from build123d import *

# Parameters (mm, degrees)
F1_DEPTH = 4.7625
F2_R     = 5.08
F4_DEPTH = 4.7635


# Not quite as in the source:
# - a length typed as a fraction of an inch, garbled in the dataset ("3 / 203.2 mm" for 3/8 in), is restored


with BuildPart() as f1:
    # F0 (on Top) → F1 (new body)
    with BuildSketch(Plane.XY):
        Polygon((124.0544550598, 72.092982788), (-155.3455449402, 72.092982788), (-155.3455449402, 27.642982788), (-76.0003953454, 27.642982788), (-37.8705449402, -29.507017212), (-37.8705449402, -80.307017212), (6.5794550598, -80.307017212), (6.5794550598, -29.507017212), (44.7093054649, 27.642982788), (124.0544550598, 27.642982788), align=None)
    extrude(amount=F1_DEPTH)

    # F2
    f2_edges = [f1.edges().sort_by_distance(p)[0] for p in [
        (-155.345545, 27.642983, 2.38125),
        (-155.345545, 72.092983, 2.38125),
        (-37.870545, -80.307017, 2.38125),
        (6.579455, -80.307017, 2.38125),
        (-76.000395, 27.642983, 2.38125),
        (-37.870545, -29.507017, 2.38125),
        (6.579455, -29.507017, 2.38125),
        (44.709305, 27.642983, 2.38125),
        (124.054455, 27.642983, 2.38125),
        (124.054455, 72.092983, 2.38125),
    ]]
    fillet(f2_edges, radius=F2_R)

    # F3 (on face) → F4 (cut, through all)
    with BuildSketch(Plane.XY.offset(4.7625)):
        with BuildLine():
            Line((106.8459550598, 54.757482788), (97.5749550598, 54.757482788))
            ThreePointArc((97.5749550598, 54.757482788), (92.6854550598, 49.867982788), (97.5749550598, 44.978482788))
            Line((97.5749550598, 44.978482788), (106.8459550598, 44.978482788))
            ThreePointArc((106.8459550598, 44.978482788), (111.7354550598, 49.867982788), (106.8459550598, 54.757482788))
        make_face()
        with BuildLine():
            Line((33.6939550598, 54.757482788), (24.4229550598, 54.757482788))
            ThreePointArc((24.4229550598, 54.757482788), (19.5334550598, 49.867982788), (24.4229550598, 44.978482788))
            Line((24.4229550598, 44.978482788), (33.6939550598, 44.978482788))
            ThreePointArc((33.6939550598, 44.978482788), (38.5834550598, 49.867982788), (33.6939550598, 54.757482788))
        make_face()
        with BuildLine():
            ThreePointArc((-10.7560449402, -63.352517212), (-15.6455449402, -58.463017212), (-20.5350449402, -63.352517212))
            Line((-20.5350449402, -63.352517212), (-20.5350449402, -72.623517212))
            ThreePointArc((-20.5350449402, -72.623517212), (-15.6455449402, -77.513017212), (-10.7560449402, -72.623517212))
            Line((-10.7560449402, -72.623517212), (-10.7560449402, -63.352517212))
        make_face()
        with BuildLine():
            Line((-10.7560449402, 0.528482788), (-10.7560449402, 9.799482788))
            ThreePointArc((-10.7560449402, 9.799482788), (-15.6455449402, 14.688982788), (-20.5350449402, 9.799482788))
            Line((-20.5350449402, 9.799482788), (-20.5350449402, 0.528482788))
            ThreePointArc((-20.5350449402, 0.528482788), (-15.6455449402, -4.361017212), (-10.7560449402, 0.528482788))
        make_face()
        with BuildLine():
            Line((-128.8660449402, 54.757482788), (-138.1370449402, 54.757482788))
            ThreePointArc((-138.1370449402, 54.757482788), (-143.0265449402, 49.867982788), (-138.1370449402, 44.978482788))
            Line((-138.1370449402, 44.978482788), (-128.8660449402, 44.978482788))
            ThreePointArc((-128.8660449402, 44.978482788), (-123.9765449402, 49.867982788), (-128.8660449402, 54.757482788))
        make_face()
        with BuildLine():
            Line((-55.7140449402, 54.757482788), (-64.9850449402, 54.757482788))
            ThreePointArc((-64.9850449402, 54.757482788), (-69.8745449402, 49.867982788), (-64.9850449402, 44.978482788))
            Line((-64.9850449402, 44.978482788), (-55.7140449402, 44.978482788))
            ThreePointArc((-55.7140449402, 44.978482788), (-50.8245449402, 49.867982788), (-55.7140449402, 54.757482788))
        make_face()
    extrude(amount=-F4_DEPTH, mode=Mode.SUBTRACT)


solid = f1.part
Can you work these out from the model? Positions are in its coordinate system, mm. A direction names the side the tool comes from. Round coordinates to 2 decimals unless told otherwise and drop trailing zeros. Write each loop counter-clockwise with the first axis right and the second up, starting at its lowest first coordinate (ties: lowest second). Pieces come first, ordered by that corner, then holes. Notation, with made-up numbers: M 7,-25 L 41,-25 A15 cw 41,-3 Z; hole C 79.5,-23.5 d9. An arc over 180 degrees is marked long. Use a Markdown table: item, result.
Item 1: For pin 1 Ø2.5 at (x, z) = (-58.5, 1.5) entering from -Y; pin 2 Ø1.4 at (x, z) = (73, 3.5) entering from -Y; pin 3 Ø8 at (x, y) = (26, 56.5) entering from -Z; pin 4 Ø1.4 at (y, z) = (6, 2.5) entering from -X, each with a flat end and sliding along its axis, tell me the tip position at first contact or that it passes through.
Found:
| item | result |
|---|---|
| pin 1 | stops at y = -0.46 |
| pin 2 | stops at y = 27.64 |
| pin 3 | stops at z = 0 |
| pin 4 | stops at x = -62.03 |
Item 2: I want a section at C-C (z = 2.8). State how many separate pieces and enclosed holes the cut face has, and give its area (3 significant figures).
Found:
| item | result |
|---|---|
| separate pieces | 1 |
| enclosed holes | 6 |
| area | 18,400 mm2 |
Item 3: I want a section at D-D (x = 84.5). List the corners of the cut face in (y, z) for me.
Found:
| item | result |
|---|---|
| outline | M 27.64,0 L 72.09,0 L 72.09,4.76 L 27.64,4.76 Z |
Item 4: I want a section at B-B (x = -60.5). List the corners of the cut face in (y, z) for me.
Found:
| item | result |
|---|---|
| outline | M 4.41,0 L 44.98,0 L 44.98,4.76 L 4.41,4.76 Z; M 54.76,0 L 72.09,0 L 72.09,4.76 L 54.76,4.76 Z |
Item 5: We'd pull the mould along X, two halves only. Please class faces 1 (the face through (25.067, -1.797, 2.348)), 2 (the face through (-50.826, 49.76, 2.415)), 3 (the face through (111.734, 49.76, 2.415)), 4 (the face through (-18, 31, 0)): released by +X, released by -X, zero draft, split by the parting line, or undercut.
Found:
| item | result |
|---|---|
| face 1 | released by +X |
| face 2 | undercut |
| face 3 | undercut |
| face 4 | zero draft |
Item 6: I want a section at A-A (y = 6.5). List the corners of the cut face in (x, z) for me, and give its area (3 significant figures).
Found:
| item | result |
|---|---|
| outline | M -61.89,0 L -20.54,0 L -20.54,4.76 L -61.89,4.76 Z; M -10.76,0 L 30.6,0 L 30.6,4.76 L -10.76,4.76 Z |
| area | 394 mm2 |
Item 7: If I drill on line 1 along X through (y, z) = (-70, 4.5); line 2 along Y through (x, z) = (-131.5, 3.3); line 3 along Y through (x, z) = (-120.5, 4.45), over which ranges is the centre line in solid material (lowest first)? Write a range as [from, to].
Found:
| item | result |
|---|---|
| line 1 | x = [-37.87, -20.54], [-10.76, 6.58] |
| line 2 | y = [27.64, 44.98], [54.76, 72.09] |
| line 3 | y = [27.64, 72.09] |
Item 8: Which directions (+Z, -Z, +X, -X, +Y, -Y) give clear straight access to the entire face, cutting with the end or side of a thin tool? Please do faces 5 (the face through (122.527, 29.092, 2.415)), 6 (the face through (38.582, 49.76, 2.415)).
Found:
| item | result |
|---|---|
| face 5 | +Z, -Z, +X, -Y |
| face 6 | +Z, -Z |
